```python
from build123d import *

# Parameters (mm, degrees)
SKETCH2_W           = 80
SKETCH2_H           = 50
BOSS_EXTRUDE1_DEPTH = 5
CUT_EXTRUDE1_DEPTH  = 10
SKETCH4_W           = 13
SKETCH4_H           = 23
CUT_EXTRUDE2_DEPTH  = 2
SKETCH6_W           = 13
SKETCH6_H           = 4.7
SKETCH6_R           = 1.5
BOSS_EXTRUDE2_DEPTH = 3
SKETCH10_W          = 80
SKETCH10_H          = 9
BOSS_EXTRUDE5_DEPTH = 10
CUT_EXTRUDE3_DEPTH  = 86.14693183
SKETCH13_W          = 10
SKETCH13_H          = 50
BOSS_EXTRUDE6_DEPTH = 12
SKETCH14_R          = 4.25
CUT_EXTRUDE4_DEPTH  = 66.76473219
SKETCH17_W          = 6.937355762
SKETCH17_H          = 20.309439226
BOSS_EXTRUDE7_DEPTH = 10
SKETCH18_W          = 5.321998735
SKETCH18_H          = 9.21217238
SKETCH18_W_2        = 3
SKETCH18_H_2        = 5.5
CUT_EXTRUDE5_DEPTH  = 53.782572882


with BuildPart() as part:
    # Sketch2 → Boss-Extrude1 (new body)
    with BuildSketch(Plane.XY):
        Rectangle(SKETCH2_W, SKETCH2_H)
    extrude(amount=BOSS_EXTRUDE1_DEPTH)

    # Sketch3 → Cut-Extrude1 (cut)
    with BuildSketch(Plane(origin=(0, 0, 0), x_dir=(-1, 0, 0), z_dir=(0, 0, -1))):
        with BuildLine():
            Line((-3, -5.196152423), (-3, -7.523942422))
            ThreePointArc((-3, -7.523942422), (0, -10.523942422), (3, -7.523942422))
            Line((3, -7.523942422), (3, -5.196152423))
            ThreePointArc((3, -5.196152423), (0, 6), (-3, -5.196152423))
        make_face()
    extrude(amount=-CUT_EXTRUDE1_DEPTH, mode=Mode.SUBTRACT)

    # Sketch4 → Cut-Extrude2 (cut)
    with BuildSketch(Plane(origin=(0, 0, 0), x_dir=(-1, 0, 0), z_dir=(0, 0, -1))):
        with Locations((0, -5.5)):
            Rectangle(SKETCH4_W, SKETCH4_H)
    extrude(amount=-CUT_EXTRUDE2_DEPTH, mode=Mode.SUBTRACT)

    # Sketch6 → Boss-Extrude2 (add)
    # profile 1 of 2: a face of its own
    with BuildSketch(Plane(origin=(0, 0, 0), x_dir=(-1, 0, 0), z_dir=(0, 0, -1))):
        with Locations((0, -19.35)):
            Rectangle(SKETCH6_W, SKETCH6_H)
        with Locations((0, -19.5)):
            Circle(SKETCH6_R, mode=Mode.SUBTRACT)
    # profile 2 of 2: a face of its own
    with BuildSketch(Plane(origin=(0, 0, 0), x_dir=(-1, 0, 0), z_dir=(0, 0, -1))):
        with Locations((0, 8.35)):
            Rectangle(SKETCH6_W, SKETCH6_H)
        with Locations(Location((0, 8.5, 0), (0, 0, 180))):
            Circle(SKETCH6_R, mode=Mode.SUBTRACT)
    extrude(amount=BOSS_EXTRUDE2_DEPTH)

    # Sketch10 → Boss-Extrude5 (add)
    with BuildSketch(Plane.XY.offset(5)):
        with Locations((0, 20.5)):
            Rectangle(SKETCH10_W, SKETCH10_H)
        with Locations((0, -20.5)):
            Rectangle(SKETCH10_W, SKETCH10_H)
    extrude(amount=BOSS_EXTRUDE5_DEPTH)

    # Sketch11 → Cut-Extrude3 (cut, through all)
    with BuildSketch(Plane(origin=(40, 0, 0), x_dir=(0, 0, -1), z_dir=(1, 0, 0))):
        Polygon((-11.279093119, 16), (-11.279093119, 17.27), (-12.551885325, 18.542792206), (-12.551885325, 21.332792206), (-5.701885325, 21.332792206), (-5.701885325, 18.542792206), (-6.969093119, 17.27), (-6.969093119, 16), align=None)
        Polygon((-11.279093119, -16), (-6.969093119, -16), (-6.969093119, -17.27), (-5.701885325, -18.542792206), (-5.701885325, -21.332792206), (-12.551885325, -21.332792206), (-12.551885325, -18.542792206), (-11.279093119, -17.27), align=None)
    extrude(amount=-CUT_EXTRUDE3_DEPTH, mode=Mode.SUBTRACT)

    # Sketch13 → Boss-Extrude6 (add)
    with BuildSketch(Plane(origin=(0, 0, 0), x_dir=(-1, 0, 0), z_dir=(0, 0, -1))):
        with Locations((-21, 0)):
            Rectangle(SKETCH13_W, SKETCH13_H)
        with Locations((21, 0)):
            Rectangle(SKETCH13_W, SKETCH13_H)
    extrude(amount=BOSS_EXTRUDE6_DEPTH)

    # Sketch14 → Cut-Extrude4 (cut, through all)
    with BuildSketch(Plane(origin=(0, 25, 0), x_dir=(1, 0, 0), z_dir=(0, 1, 0))):
        with Locations(Location((-21, 6, 0), (0, 0, 270))):
            Circle(SKETCH14_R)
        with Locations(Location((21, 6, 0), (0, 0, 90))):
            Circle(SKETCH14_R)
    extrude(amount=-CUT_EXTRUDE4_DEPTH, mode=Mode.SUBTRACT)

    # Sketch17 → Boss-Extrude7 (add)
    with BuildSketch(Plane(origin=(0, 0, 0), x_dir=(-1, 0, 0), z_dir=(0, 0, -1))):
        with Locations((10.005383819, -4.154719613)):
            Rectangle(SKETCH17_W, SKETCH17_H)
        with Locations((-10.005383819, -4.154719613)):
            Rectangle(SKETCH17_W, SKETCH17_H)
    extrude(amount=BOSS_EXTRUDE7_DEPTH)

    # Sketch18 → Cut-Extrude5 (cut, through all)
    with BuildSketch(Plane(origin=(0, 6, 0), x_dir=(1, 0, 0), z_dir=(0, 1, 0))):
        with Locations((10.030343861, 4.611072031)):
            Rectangle(SKETCH18_W, SKETCH18_H)
        with Locations((-10.810103866, 5.140004806)):
            Rectangle(SKETCH18_W_2, SKETCH18_H_2)
    extrude(amount=-CUT_EXTRUDE5_DEPTH, mode=Mode.SUBTRACT)


solid = part.part
```
Here's how the part is built. I have some questions about the finished solid (model axes, mm). A direction names the side the tool comes from. Coordinates: 2 decimals unless noted, no trailing zeros. Write each loop counter-clockwise with the first axis right and the second up, starting at its lowest first coordinate (ties: lowest second). Pieces come first, ordered by that corner, then holes. Notation, with made-up numbers: (23, 46) - (49, 46) arc R26 ccw to (49, 60) - close; hole circle Ø7 at (77.5, 83.25). An arc over 180 degrees is marked (long way). One line per item, written item: value.
1) Suppose I cut it at B-B on z = -6. State how many separate pieces and enclosed holes the cut face has, and give its area (3 significant figures).
Model answer:
separate pieces: 8
enclosed holes: 0
area: 263 mm²
2) We'd pull the mould along X, two halves only. Please class faces 6 (the flat face through (-6.537, -4, -5)), 7 (the flat face through (-1, -16, 13)), 8 (the flat face through (-6.5, -6, 1)): pulls with the +X half, pulls with the -X half, needs draft (parallel to the pull), parting line crosses it, or undercut.
Model answer:
face 6: undercut
face 7: needs draft
face 8: undercut
3) On a 3-axis mill with a long thin cutter (end or side, diameter ignored), from which of +Z, -Z, +X, -X, +Y, -Y can I reach the whole of each face in a straight line? I mean faces 1 (the flat face through (1, -21.333, 9)), 2 (the flat face through (10, -4, -9.217)), 3 (the flat face through (0, -19, 0)), 4 (the flat face through (33, 0, 0)), 5 (the flat face through (-13.474, -4, -5)). Say none if no direction works.
Model answer:
face 1: +X, -X
face 2: +Y, -Y
face 3: -Z
face 4: -Z, +X, +Y, -Y
face 5: -Z, +Y, -Y
4) I'm going to push flat-ended pins straight in: P1, Ø8, axis at y = -7.5, z = -4.5, coming from the +X side; P2, Ø0.9, axis at x = -11, y = -8.5, coming from the +Z side; P3, Ø3.5, axis at x = 3, z = -2, coming from the -Y side; P4, Ø11, axis at x = 0, y = 0, coming from the +Z side. Where does each tip first touch, or does it pass through?
Model answer:
P1: stops at x = 26
P2: stops at z = 5
P3: stops at y = -21.7
P4: passes through
5) Suppose I cut it at D-D on z = 10. Write out the boundary of the cut face in (x, y), and give its area (3 significant figures).
Model answer:
outline: (-40, -25) - (40, -25) - (40, -21.33) - (-40, -21.33) - close; (-40, 21.33) - (40, 21.33) - (40, 25) - (-40, 25) - close
area: 587 mm²
6) Suppose I cut it at A-A on x = 21. Write out the boundary of the cut face in (y, z).
Model answer:
outline: (-25, -12) - (25, -12) - (25, -10.25) - (-25, -10.25) - close; (-25, -1.75) - (25, -1.75) - (25, 15) - (16, 15) - (16, 11.28) - (17.27, 11.28) - (18.54, 12.55) - (21.33, 12.55) - (21.33, 5.7) - (18.54, 5.7) - (17.27, 6.97) - (16, 6.97) - (16, 5) - (-16, 5) - (-16, 6.97) - (-17.27, 6.97) - (-18.54, 5.7) - (-21.33, 5.7) - (-21.33, 12.55) - (-18.54, 12.55) - (-17.27, 11.28) - (-16, 11.28) - (-16, 15) - (-25, 15) - close
7) I need wall thicknesses on line 1 along Y through (x, z) = (0, -1.5); line 2 along X through (y, z) = (8.5, -1.3); line 3 along X through (y, z) = (10, -6). Which ranges of each line are inside material? Lowest first, please.
Model answer:
line 1: y = -21.7 to -21, -18 to -17, 6 to 7, 10 to 10.7
line 2: x = -26 to -16, -6.5 to -1.5, 1.5 to 6.5, 16 to 26
line 3: x = -26 to -25.25, -16.75 to -16, 16 to 16.75, 25.25 to 26
8) Suppose I cut it at C-C on y = 8.5. Write out the boundary of the cut face in (x, z).
Model answer:
outline: (-40, 0) - (-26, 0) - (-26, -12) - (-16, -12) - (-16, 0) - (-6.5, 0) - (-6.5, -3) - (-1.5, -3) - (-1.5, 0) - (1.5, 0) - (1.5, -3) - (6.5, -3) - (6.5, 0) - (16, 0) - (16, -12) - (26, -12) - (26, 0) - (40, 0) - (40, 5) - (-40, 5) - close; hole circle Ø8.5 at (-21, -6); hole circle Ø8.5 at (21, -6)
